from build123d import *

# Parameters (mm, degrees)
ESBO_O1_R                     = 35
ESBO_O1_R_2                   = 32.5
RESSALTO_EXTRUS_O1_DEPTH      = 8
RESSALTO_EXTRUS_O2_START      = -3
ESBO_O2_R                     = 32.5
RESSALTO_EXTRUS_O2_DEPTH      = 3
ESBO_O3_R                     = 2.5
CORTE_EXTRUS_O1_DEPTH         = 3
RESSALTO_EXTRUS_O3_DEPTH      = 5
RESSALTO_EXTRUS_O3_DEPTH_BACK = 3
ESBO_O4_R                     = 37
ESBO_O4_R_2                   = 35
ESBO_O5_W                     = 1.8
ESBO_O5_H                     = 3
ESBO_O6_R                     = 12.55
RESSALTO_EXTRUS_O4_DEPTH      = 5
CORTE_EXTRUS_O2_DEPTH         = 53.933921071
CORTE_EXTRUS_O2_DEPTH_BACK    = 53.933921071
ESBO_O7_R                     = 7.55
RESSALTO_EXTRUS_O5_START      = -8
ESBO_O8_R                     = 37
ESBO_O8_R_2                   = 32.5
RESSALTO_EXTRUS_O5_DEPTH      = 8
ESBO_O9_R                     = 37
ESBO_O9_R_2                   = 33.5
CORTE_EXTRUS_O8_DEPTH         = 1.5
CORTE_EXTRUS_O9_START         = -1.5
ESBO_O12_R                    = 37
ESBO_O12_R_2                  = 33.5
CORTE_EXTRUS_O9_DEPTH         = 1.5
CORTE_EXTRUS_O10_START        = -10
ESBO_O13_R                    = 37
ESBO_O13_R_2                  = 36
CORTE_EXTRUS_O10_DEPTH        = 10
ESBO_O14_R                    = 37
ESBO_O14_R_2                  = 36
RESSALTO_EXTRUS_O6_DEPTH      = 5
ESBO_O15_R                    = 12.55
CORTE_EXTRUS_O11_DEPTH        = 53.933921071
ESBO_O16_R                    = 12.55
RESSALTO_EXTRUS_O7_DEPTH      = 3
ESBO_O17_R                    = 10
RESSALTO_EXTRUS_O8_DEPTH      = 16
ESBO_O18_R                    = 3.3
CORTE_EXTRUS_O12_DEPTH        = 16
ESBO_O19_W                    = 5.95
ESBO_O19_H                    = 2.65
CORTE_EXTRUS_O13_DEPTH        = 8
CORTE_EXTRUS_O14_DEPTH        = 58.265085349
CORTE_EXTRUS_O14_DEPTH_BACK   = 58.265085349
ESBO_O21_R                    = 1.65
ESBO_O23_R                    = 37
ESBO_O23_R_2                  = 36
CORTE_EXTRUS_O15_DEPTH        = 54.798234195
ESBO_O24_R                    = 3.3
CORTE_EXTRUS_O16_DEPTH        = 55.341512677


with BuildPart() as part:
    # Esboço1 → Ressalto-extrusão1 (new body)
    with BuildSketch(Plane.XY):
        Circle(ESBO_O1_R)
        Circle(ESBO_O1_R_2, mode=Mode.SUBTRACT)
    extrude(amount=RESSALTO_EXTRUS_O1_DEPTH)

    # Esboço2 → Ressalto-extrusão2 (add)
    with BuildSketch(Plane.XY.offset(8).offset(RESSALTO_EXTRUS_O2_START)):
        Circle(ESBO_O2_R)
    extrude(amount=RESSALTO_EXTRUS_O2_DEPTH)

    # Esboço3 → Corte-extrusão1 (cut)
    with BuildSketch(Plane.XY.offset(8)):
        Circle(ESBO_O3_R)
    extrude(amount=-CORTE_EXTRUS_O1_DEPTH, mode=Mode.SUBTRACT)

    # Esboço4 → Ressalto-extrusão3 (add, two sides: drawn at the far end of the back side and taken through both)
    with BuildSketch(Plane(origin=(0, 0, 5), x_dir=(-1, 0, 0), z_dir=(0, 0, -1)).offset(-RESSALTO_EXTRUS_O3_DEPTH_BACK)):
        Circle(ESBO_O4_R)
        Circle(ESBO_O4_R_2, mode=Mode.SUBTRACT)
    extrude(amount=RESSALTO_EXTRUS_O3_DEPTH + RESSALTO_EXTRUS_O3_DEPTH_BACK)

    # Esboço5 → Corte-Revolução1 (revolve, cut)
    with BuildSketch(Plane(origin=(0, 0, 0), x_dir=(1, 0, 0), z_dir=(0, 1, 0))):
        with Locations((-36.1, -2.5)):
            Rectangle(ESBO_O5_W, ESBO_O5_H)
        with Locations((-36.1, -5.5)):
            Rectangle(ESBO_O5_W, ESBO_O5_H)
    revolve(axis=Axis((0, 0, 8), (0, 0, -1)), mode=Mode.SUBTRACT)

    # Esboço6 → Ressalto-extrusão4 (add)
    with BuildSketch(Plane(origin=(0, 0, 5), x_dir=(-1, 0, 0), z_dir=(0, 0, -1))):
        with Locations(Location((0, 0, 0), (0, 0, 180))):
            Circle(ESBO_O6_R)
    extrude(amount=RESSALTO_EXTRUS_O4_DEPTH)

    # Esboço7 → Corte-extrusão2 (cut, two sides: drawn at the far end of the back side and taken through both)
    with BuildSketch(Plane(origin=(0, 0, 0), x_dir=(-1, 0, 0), z_dir=(0, 0, -1)).offset(-CORTE_EXTRUS_O2_DEPTH_BACK)):
        Circle(ESBO_O7_R)
    extrude(amount=CORTE_EXTRUS_O2_DEPTH + CORTE_EXTRUS_O2_DEPTH_BACK, mode=Mode.SUBTRACT)

    # Esboço8 → Ressalto-extrusão5 (add)
    with BuildSketch(Plane.XY.offset(8).offset(RESSALTO_EXTRUS_O5_START)):
        with Locations(Location((0, 0, 0), (0, 0, 180))):
            Circle(ESBO_O8_R)
        Circle(ESBO_O8_R_2, mode=Mode.SUBTRACT)
    extrude(amount=RESSALTO_EXTRUS_O5_DEPTH)

    # Esboço9 → Corte-extrusão8 (cut)
    with BuildSketch(Plane.XY.offset(8)):
        with Locations(Location((0, 0, 0), (0, 0, 180))):
            Circle(ESBO_O9_R)
        Circle(ESBO_O9_R_2, mode=Mode.SUBTRACT)
    extrude(amount=-CORTE_EXTRUS_O8_DEPTH, mode=Mode.SUBTRACT)

    # Esboço12 → Corte-extrusão9 (cut)
    with BuildSketch(Plane(origin=(0, 0, 0), x_dir=(-1, 0, 0), z_dir=(0, 0, -1)).offset(CORTE_EXTRUS_O9_START)):
        Circle(ESBO_O12_R)
        with Locations(Location((0, 0, 0), (0, 0, 180))):
            Circle(ESBO_O12_R_2, mode=Mode.SUBTRACT)
    extrude(amount=CORTE_EXTRUS_O9_DEPTH, mode=Mode.SUBTRACT)

    # Esboço13 → Corte-extrusão10 (cut)
    with BuildSketch(Plane(origin=(0, 0, 1.5), x_dir=(-1, 0, 0), z_dir=(0, 0, -1)).offset(CORTE_EXTRUS_O10_START)):
        Circle(ESBO_O13_R)
        Circle(ESBO_O13_R_2, mode=Mode.SUBTRACT)
    extrude(amount=CORTE_EXTRUS_O10_DEPTH, mode=Mode.SUBTRACT)

    # Esboço14 → Ressalto-extrusão6 (add)
    with BuildSketch(Plane.XY.offset(6.5)):
        Circle(ESBO_O14_R)
        Circle(ESBO_O14_R_2, mode=Mode.SUBTRACT)
    extrude(amount=-RESSALTO_EXTRUS_O6_DEPTH)

    # Esboço15 → Corte-extrusão11 (cut, through all)
    with BuildSketch(Plane(origin=(0, 0, 0), x_dir=(-1, 0, 0), z_dir=(0, 0, -1))):
        Circle(ESBO_O15_R)
    extrude(amount=-CORTE_EXTRUS_O11_DEPTH, mode=Mode.SUBTRACT)

    # Esboço16 → Ressalto-extrusão7 (add, through all)
    with BuildSketch(Plane(origin=(0, 0, 5), x_dir=(-1, 0, 0), z_dir=(0, 0, -1))):
        Circle(ESBO_O16_R)
    extrude(amount=-RESSALTO_EXTRUS_O7_DEPTH)

    # Esboço17 → Ressalto-extrusão8 (add)
    with BuildSketch(Plane(origin=(0, 0, 5), x_dir=(-1, 0, 0), z_dir=(0, 0, -1))):
        with Locations(Location((0, 0, 0), (0, 0, 180))):
            Circle(ESBO_O17_R)
    extrude(amount=RESSALTO_EXTRUS_O8_DEPTH)

    # Esboço18 → Corte-extrusão12 (cut)
    with BuildSketch(Plane(origin=(0, 0, -11), x_dir=(-1, 0, 0), z_dir=(0, 0, -1))):
        Circle(ESBO_O18_R)
    extrude(amount=-CORTE_EXTRUS_O12_DEPTH, mode=Mode.SUBTRACT)

    # Esboço19 → Corte-extrusão13 (cut)
    with BuildSketch(Plane(origin=(0, 0, -11), x_dir=(-1, 0, 0), z_dir=(0, 0, -1))):
        with Locations((0, -6.625)):
            Rectangle(ESBO_O19_W, ESBO_O19_H)
        with Locations((0, 6.625)):
            Rectangle(ESBO_O19_W, ESBO_O19_H)
    extrude(amount=-CORTE_EXTRUS_O13_DEPTH, mode=Mode.SUBTRACT)

    # Esboço21 → Corte-extrusão14 (cut, two sides: drawn at the far end of the back side and taken through both)
    with BuildSketch(Plane(origin=(0, 5.3, 0), x_dir=(1, 0, 0), z_dir=(0, 1, 0)).offset(-CORTE_EXTRUS_O14_DEPTH_BACK)):
        with Locations(Location((0, 6.85, 0), (0, 0, 180))):
            Circle(ESBO_O21_R)
    extrude(amount=CORTE_EXTRUS_O14_DEPTH + CORTE_EXTRUS_O14_DEPTH_BACK, mode=Mode.SUBTRACT)

    # Esboço23 → Corte-extrusão15 (cut, through all)
    with BuildSketch(Plane(origin=(0, 0, 1.5), x_dir=(-1, 0, 0), z_dir=(0, 0, -1))):
        Circle(ESBO_O23_R)
        Circle(ESBO_O23_R_2, mode=Mode.SUBTRACT)
    extrude(amount=-CORTE_EXTRUS_O15_DEPTH, mode=Mode.SUBTRACT)

    # Esboço24 → Corte-extrusão16 (cut, through all)
    with BuildSketch(Plane(origin=(0, 0, -11), x_dir=(-1, 0, 0), z_dir=(0, 0, -1))):
        Circle(ESBO_O24_R)
    extrude(amount=-CORTE_EXTRUS_O16_DEPTH, mode=Mode.SUBTRACT)


solid = part.part
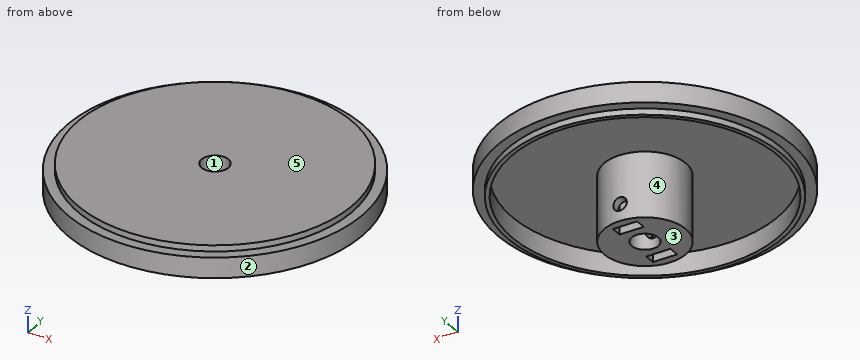
Work out the finished part from the listing and answer in its coordinate system (mm). Face numbers are marked on the shaded views. A direction names the side the tool comes from. Round coordinates to 2 decimals unless told otherwise and drop trailing zeros. Loops run counter-clockwise (first coordinate to the right, second up) from the corner with the lowest first, then second, coordinate; pieces in that order, holes last. Notation, with made-up numbers: (18, 83) - (39, 83) arc R18 cw to (39, 103) - close; hole circle Ø4 at (23.5, 28.5). An arc over 180 degrees is marked (long way). One line per item, written item: value.
Q1. Find section A-A on y = 0. Give the vertices of the cut face in (x, z), and give its area (3 significant figures).
Check values:
outline: (-36, 1.5) - (-33.5, 1.5) - (-33.5, 0) - (-32.5, 0) - (-32.5, 5) - (-10, 5) - (-10, -11) - (-3.3, -11) - (-3.3, 8) - (-33.5, 8) - (-33.5, 6.5) - (-36, 6.5) - close; (3.3, -11) - (10, -11) - (10, 5) - (32.5, 5) - (32.5, 0) - (33.5, 0) - (33.5, 1.5) - (36, 1.5) - (36, 6.5) - (33.5, 6.5) - (33.5, 8) - (3.3, 8) - close
area: 431 mm2
Q2. The mould has two halves that part along Y. Classify the marked faces 1, 2 and 3: +Y half, -Y half, draft (parallel to the pull), parting line (faces both ways), or undercut.
Check values:
face 1: undercut
face 2: parting line
face 3: draft
Q3. Each of these flat-tipped pins is pushed along its axis until it touches: pin 1 Ø0.8 at (y, z) = (7, -6.5) entering from -X; pin 2 Ø4.5 at (x, z) = (0, -6.85) entering from -Y; pin 3 Ø3 at (x, z) = (-6.5, 2) entering from -Y; pin 4 Ø2 at (x, y) = (1, 7) entering from -Z. Where does it stop, or does it pass through?
Check values:
pin 1: x = -7.51
pin 2: y = -10
pin 3: y = -35.65
pin 4: z = -11
Q4. Straight lines are drawn through the part: probe 1 along Y at (x, z) = (0, 3.5); probe 2 along Y at (x, z) = (0, 1.35); probe 3 along Z at (x, y) = (0, -8.4). For each, find the intervals that lie inside material, in ascending order.
Check values:
probe 1: -36 to -32.5, -10 to -3.3, 3.3 to 10, 32.5 to 36
probe 2: -33.5 to -32.5, -10 to -3.3, 3.3 to 10, 32.5 to 33.5
probe 3: -11 to -8.5, -5.2 to 8
Q5. Find section C-C on x = -27.5. Give the vertices of the cut face in (y, z).
Check values:
outline: (-23.23, 1.5) - (-19.13, 1.5) - (-19.13, 0) - (-17.32, 0) - (-17.32, 5) - (17.32, 5) - (17.32, 0) - (19.13, 0) - (19.13, 1.5) - (23.23, 1.5) - (23.23, 6.5) - (19.13, 6.5) - (19.13, 8) - (-19.13, 8) - (-19.13, 6.5) - (-23.23, 6.5) - close
Q6. For the marked faces 4 and 5, determine the directions among +Z, -Z, +X, -X, +Y, -Y from which every point of the face is accessible in a straight line to the end or side of a thin tool.
Check values:
face 4: -Z
face 5: +Z, +X, -X, +Y, -Y
Q7. Find section B-B on z = -9.5. Give the vertices of the cut face in (x, y) (3 decimals).
Check values:
outline: circle Ø20 at (0, 0); hole circle Ø6.6 at (0, 0); hole (-2.975, -7.95) - (2.975, -7.95) - (2.975, -5.3) - (-2.975, -5.3) - close; hole (-2.975, 5.3) - (2.975, 5.3) - (2.975, 7.95) - (-2.975, 7.95) - close
Q8. Find section D-D on z = -1.75. Give the vertices of the cut face in (x, y), and give its area (3 significant figures).
Check values:
outline: circle Ø20 at (0, 0); hole circle Ø6.6 at (0, 0)
area: 280 mm2
